Part model, mm, in its own coordinate system. A direction names the side the tool comes from. Round coordinates to 2 decimals unless told otherwise and drop trailing zeros. Loops run counter-clockwise (first coordinate to the right, second up) from the corner with the lowest first, then second, coordinate; pieces in that order, holes last. Notation, with made-up numbers: (-9, -14) -> (9, -14) arc R30 cw to (9, 19) -> close; hole circle Ø10 at (-17, -15.5). An arc over 180 degrees is marked (long way). Answer as CSV lines item,"result".
from build123d import *

# Parameters (mm, degrees)
F1_DEPTH = 2.5
F2_R     = 5
F3_DEPTH = 1


with BuildPart() as f1:
    # F0 (on Front) → F1 (new body)
    with BuildSketch(Plane.XZ):
        Polygon((3.207181, 5.555), (-3.207181, 5.555), (-6.414361, 0), (-3.207181, -5.555), (3.207181, -5.555), (6.414361, 0), align=None)
    extrude(amount=F1_DEPTH)

    # F2 (on Front) → F3 (join)
    with BuildSketch(Plane.XZ):
        Circle(F2_R)
    extrude(amount=-F3_DEPTH)


solid = f1.part
Q1. Which spindle directions (+Z, -Z, +X, -X, +Y, -Y) get a long thin tool onto all of the face, cutting with end or side? Do faces 1 (the face through (0, -2.5, 0)), 2 (the face through (5, 0, 2)). Say none if no direction does.
Geometry results:
face 1,"+Z, -Z, +X, -X, -Y"
face 2,"+Y"
Q2. Saw through at C-C, the plane y = 0.2. Write the cut outline in (x, z).
Geometry results:
outline,"circle Ø10 at (0, 0)"
Q3. Saw through at A-A, the plane x = 0. Write the cut outline in (y, z) (3 decimals).
Geometry results:
outline,"(-2.5, -5.555) -> (0, -5.555) -> (0, -5) -> (1, -5) -> (1, 5) -> (0, 5) -> (0, 5.555) -> (-2.5, 5.555) -> close"
Q4. Drill centre lines: line 1 along Y through (x, z) = (-5.25, -1.5); line 2 along Z through (x, y) = (-2.25, 0.2); line 3 along Z through (x, y) = (-0.75, 0.45). Where is each one in solid material? Low to high.
Geometry results:
line 1,"-2.5 to 0"
line 2,"-4.47 to 4.47"
line 3,"-4.94 to 4.94"
Q5. Saw through at B-B, the plane z = -2.25. Write the cut outline in (x, y).
Geometry results:
outline,"(-5.12, -2.5) -> (5.12, -2.5) -> (5.12, 0) -> (4.47, 0) -> (4.47, 1) -> (-4.47, 1) -> (-4.47, 0) -> (-5.12, 0) -> close"
